Geometry check sheet. Reference: the model listing, model coordinates, mm. A direction names the side the tool comes from. Give positions to 0.01 mm unless a question says otherwise; leave off trailing zeros. Write each loop counter-clockwise with the first axis right and the second up, starting at its lowest first coordinate (ties: lowest second). Pieces come first, ordered by that corner, then holes.
(1) Cross-section at C-C (z = -404). Record the boundary of the cut face in (x, y), and give its area (3 significant figures).
(2) Cross-section at A-A (y = 9). Record the boundary of the cut face in (x, z).
(3) Cross-section at B-B (x = -241). Record the boundary of the cut face in (y, z), and give its area (3 significant figures).
(4) Mould release check, pull along X, two halves, no side actions. Record for faces 4 (the flat face through (-48, 0, 582)), 5 (the flat face through (-572, 20, 8)), 6 (the flat face through (610, 20, 9)), 7 (the flat face through (-48, 38, 583)): +X half, -X half, draft (parallel to the pull), parting line (faces both ways), or undercut.
(5) Thickness scan on line 1 along Z through (x, y) = (247, 35). Record the ranges inside material, lowest first.
(6) Tool access check on faces 1 (the flat face through (-8, 20, -572)), 2 (the flat face through (-9, 20, 610)), 3 (the flat face through (-8, 20, 570)). Record the directions out of +Z, -Z, +X, -X, +Y, -Y that give a thin tool (end or side, any length) a straight path to the whole face; none if there is none.
```python
from build123d import *

# Parameters (mm, degrees)
SKETCH1_W           = 1220
SKETCH1_H           = 1220
SKETCH1_W_2         = 1140
SKETCH1_H_2         = 1140
BOSS_EXTRUDE1_DEPTH = 40
SHELL1_START        = 2
SHELL1_OUTLINE_W    = 1216
SHELL1_OUTLINE_H    = 1216
SHELL1_OUTLINE_W_2  = 1144
SHELL1_OUTLINE_H_2  = 1144
SHELL1_DEPTH        = 36
FILLET1_R           = 3


# Read off the part's stored shape, not the designer's step: Shell1
with BuildPart() as part:
    # Sketch1 → Boss-Extrude1 (new body)
    with BuildSketch(Plane(origin=(0, 0, 0), x_dir=(1, 0, 0), z_dir=(0, 1, 0))):
        Rectangle(SKETCH1_W, SKETCH1_H)
        Rectangle(SKETCH1_W_2, SKETCH1_H_2, mode=Mode.SUBTRACT)
    extrude(amount=BOSS_EXTRUDE1_DEPTH)

    # Shell1 outline → Shell1 (cut)
    with BuildSketch(Plane(origin=(0, 0, 0), x_dir=(1, 0, 0), z_dir=(0, 1, 0)).offset(SHELL1_START)):
        Rectangle(SHELL1_OUTLINE_W, SHELL1_OUTLINE_H)
        Rectangle(SHELL1_OUTLINE_W_2, SHELL1_OUTLINE_H_2, mode=Mode.SUBTRACT)
    extrude(amount=SHELL1_DEPTH, mode=Mode.SUBTRACT)

    # Fillet1
    fillet1_edges = [part.edges().sort_by_distance(p)[0] for p in [
        (-610, 40, 0),
        (0, 40, 610),
        (570, 0, 0),
        (0, 0, -570),
        (-570, 0, 0),
        (0, 0, 570),
        (570, 40, 0),
        (0, 40, -570),
        (-570, 40, 0),
        (0, 40, 570),
        (610, 40, 0),
        (0, 0, 610),
        (-610, 0, 0),
        (0, 0, -610),
        (610, 0, 0),
        (0, 40, -610),
    ]]
    fillet(fillet1_edges, radius=FILLET1_R)


solid = part.part
```
Reply:
1. outline: (-610, 3) arc R3 ccw to (-607, 0) - (-573, 0) arc R3 ccw to (-570, 3) - (-570, 37) arc R3 ccw to (-573, 40) - (-607, 40) arc R3 ccw to (-610, 37) - close; (570, 3) arc R3 ccw to (573, 0) - (607, 0) arc R3 ccw to (610, 3) - (610, 37) arc R3 ccw to (607, 40) - (573, 40) arc R3 ccw to (570, 37) - close; hole (-608, 2) - (-572, 2) - (-572, 38) - (-608, 38) - close; hole (572, 2) - (608, 2) - (608, 38) - (572, 38) - close
1. area: 593 mm2
2. outline: (-610, -610) - (610, -610) - (610, 610) - (-610, 610) - close; (-572, -572) - (572, -572) - (572, 572) - (-572, 572) - close; hole (-608, -608) - (608, -608) - (608, 608) - (-608, 608) - close; hole (-570, -570) - (570, -570) - (570, 570) - (-570, 570) - close
3. outline: (0, -607) arc R3 ccw to (3, -610) - (37, -610) arc R3 ccw to (40, -607) - (40, -573) arc R3 ccw to (37, -570) - (3, -570) arc R3 ccw to (0, -573) - close; (0, 573) arc R3 ccw to (3, 570) - (37, 570) arc R3 ccw to (40, 573) - (40, 607) arc R3 ccw to (37, 610) - (3, 610) arc R3 ccw to (0, 607) - close; hole (2, -608) - (38, -608) - (38, -572) - (2, -572) - close; hole (2, 572) - (38, 572) - (38, 608) - (2, 608) - close
3. area: 593 mm2
4. face 4: draft
4. face 5: undercut
4. face 6: +X half
4. face 7: undercut
5. line 1: z = -610 to -608, -572 to -570, 570 to 572, 608 to 610
6. face 1: none
6. face 2: +Z, +X, -X, +Y, -Y
6. face 3: +Y, -Y
